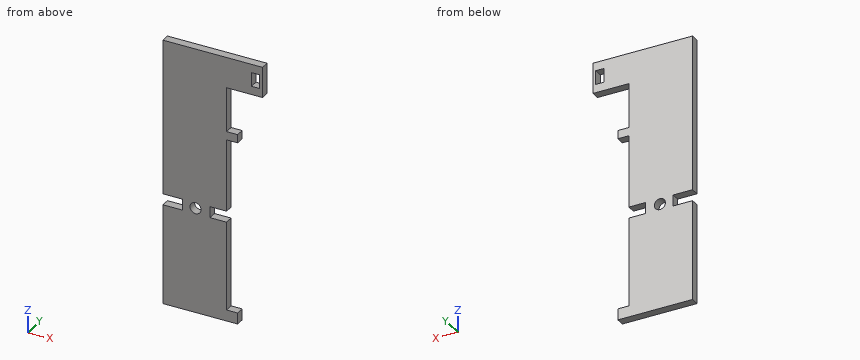
```python
from build123d import *

# Parameters (mm, degrees)
F1_DEPTH = 3
F2_R     = 2
F2_W     = 3
F2_H     = 5
F2_W_2   = 7
F2_H_2   = 4
F3_DEPTH = 25


with BuildPart() as f1:
    # F0 (on Front) → F1 (new body)
    with BuildSketch(Plane.XZ):
        Polygon((20.970293, 38.793614), (-15.029707, 38.793614), (-15.029707, -57.206386), (11.970293, -57.206386), (11.970293, -53.206386), (7.970293, -53.206386), (7.970293, -21.206386), (1.970293, -21.206386), (1.970293, -17.206386), (7.970293, -17.206386), (7.970293, 8.793614), (11.970293, 8.793614), (11.970293, 11.793614), (7.970293, 11.793614), (7.970293, 27.793614), (20.970293, 27.793614), align=None)
    extrude(amount=F1_DEPTH)

    # F2 (on face) → F3 (cut)
    with BuildSketch(Plane.XZ.offset(3)):
        with Locations((-3.233321, -19.206386)):
            Circle(F2_R)
        with Locations((18.470293, 33.293614)):
            Rectangle(F2_W, F2_H)
        with Locations((-11.529707, -19.206386)):
            Rectangle(F2_W_2, F2_H_2)
    extrude(amount=-F3_DEPTH, mode=Mode.SUBTRACT)


solid = f1.part
```
Model file for the job. Use its own axes, mm. Round coordinates to 2 decimals unless told otherwise and drop trailing zeros. Loops run counter-clockwise (first coordinate to the right, second up) from the corner with the lowest first, then second, coordinate; pieces in that order, holes last. Notation, with made-up numbers: M 74.5,-16.5 L 82.5,-16.5 A26 ccw 82.5,16.5 Z; hole C -35.75,83.5 d2. An arc over 180 degrees is marked long. Put each result on its own line as item: value. Start each with the question number.
Item 1: Drill centre lines: line 1 along Z through (x, y) = (6.5, -1.15); line 2 along X through (y, z) = (-2.1, 33.5); line 3 along X through (y, z) = (-0.55, -29). Where is each one in solid material? Low to high.
Item 2: Cut at B-B (x = 10). List the corners of the cut face in (y, z).
Item 3: Drop flat-ended pins along their axis: P1, Ø1.5, axis at y = -1, z = -10, coming from the +X side; P2, Ø0.9, axis at y = -2, z = -55.5, coming from the +X side; P3, Ø0.9, axis at y = -2, z = -18.5, coming from the +X side. Give the stop position or say it passes through.
Item 4: Cut at A-A (x = -10). List the corners of the cut face in (y, z), then the cut area to 3 significant figures.
Item 5: Cut at C-C (y = -1.6). List the corners of the cut face in (x, z), then the cut area to 3 significant figures.
Item 6: Cut at D-D (z = 21). List the corners of the cut face in (x, y).
Answer block:
1. line 1: -57.21 to -21.21, -17.21 to 38.79
1. line 2: -15.03 to 16.97, 19.97 to 20.97
1. line 3: -15.03 to 7.97
2. outline: M -3,-57.21 L 0,-57.21 L 0,-53.21 L -3,-53.21 Z; M -3,8.79 L 0,8.79 L 0,11.79 L -3,11.79 Z; M -3,27.79 L 0,27.79 L 0,38.79 L -3,38.79 Z
3. P1: x = 7.97
3. P2: x = 11.97
3. P3: x = 1.97
4. outline: M -3,-57.21 L 0,-57.21 L 0,-21.21 L -3,-21.21 Z; M -3,-17.21 L 0,-17.21 L 0,38.79 L -3,38.79 Z
4. area: 276 mm2
5. outline: M -15.03,-57.21 L 11.97,-57.21 L 11.97,-53.21 L 7.97,-53.21 L 7.97,-21.21 L 1.97,-21.21 L 1.97,-17.21 L 7.97,-17.21 L 7.97,8.79 L 11.97,8.79 L 11.97,11.79 L 7.97,11.79 L 7.97,27.79 L 20.97,27.79 L 20.97,38.79 L -15.03,38.79 L -15.03,-17.21 L -8.03,-17.21 L -8.03,-21.21 L -15.03,-21.21 Z; hole C -3.23,-19.21 d4; hole M 16.97,30.79 L 19.97,30.79 L 19.97,35.79 L 16.97,35.79 Z
5. area: 2,300 mm2
6. outline: M -15.03,-3 L 7.97,-3 L 7.97,0 L -15.03,0 Z
